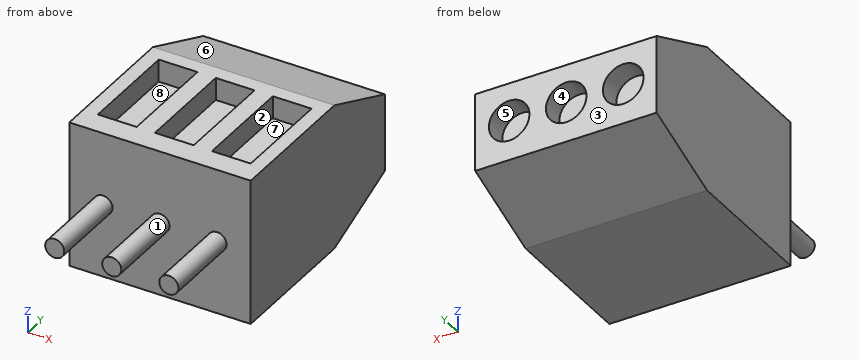
Autodesk Inventor part; units mm, degrees
ref_plane "YZ Plane" through (0, 0, 0) normal (1, 0, 0) x (0, 1, 0)
ref_plane "XZ Plane" through (0, 0, 0) normal (0, 1, 0) x (-1, 0, 0)
ref_plane "XY Plane" through (0, 0, 0) normal (0, 0, 1) x (1, 0, 0)
sketch "Sketch1" plane through (0, 0, 0) normal (1, 0, 0) x (0, 1, 0)
  line L0 (0, 3.25) -> (10, 3.25)
  line L1 (10, 3.25) -> (10, -3.25)
  line L2 (10, -3.25) -> (0, -3.25)
  line L3 (0, -3.25) -> (0, 3.25)
  line L4 (10, 1.6898) -> (6.2365, 3.25)
  line L5 (10, -1.7859) -> (6.2365, -3.25)
  point P0 (0, 0)
  dimension "d0" = 10
  dimension "d1" = 6.5
  dimension "d2" = 3.25
  dimension "d3" = 0
extrude "Extrusion1" add sketch "Sketch1" along normal mid plane 8.08 contours L0 L4 L1 L5 L2 L3
sketch "Sketch2" plane through (-4.04, 0, -3.25) normal (0, -1, 0) x (1, 0, 0)
  circle A0 centre (1.5, 3.25) radius 0.425
  line L0 (0, 0) -> (0, 6.5)
  point P0 (4.04, 3.25)
  dimension "d7" = 0.85
  dimension "d12" = 1.5
extrude "Extrusion2" add sketch "Sketch2" along normal blind 3.6
sketch "Sketch3" plane through (-4.04, 10, 1.6898) normal (0, 1, 0) x (1, 0, 0)
  circle A0 centre (1.4879, 1.6898) radius 0.904
  point P0 (4.04, 1.6898)
extrude "Extrusion3" cut sketch "Sketch3" against normal blind 1
sketch "Sketch4" plane through (-4.04, 0, 3.25) normal (0, 0, 1) x (1, 0, 0)
  line L0 (0.648, 5.5866) -> (2.3749, 5.5866)
  line L1 (2.3749, 5.5866) -> (2.3749, 1.0456)
  line L2 (2.3749, 1.0456) -> (0.648, 1.0456)
  line L3 (0.648, 1.0456) -> (0.648, 5.5866)
  point P0 (4.04, 0)
extrude "Extrusion4" cut sketch "Sketch4" against normal blind 1
pattern_linear "Rectangular Pattern1" count 3 spacing 2.54 along (1, 0, 0) of "Extrusion4", "Extrusion3", "Extrusion2"
properties part number "Screw_Terminal_3Pos"
CAD build for the part. Positions are in the model's coordinates, mm. Face numbers are marked on the shaded views. A direction names the side the tool comes from. Round coordinates to 2 decimals unless told otherwise and drop trailing zeros. Order: outer loops, then holes, each group sorted by start corner. A loop starts at its lowest first (then second) coordinate and runs counter-clockwise, first axis right, second up.
Q1. Slice it at A-A (z = 0). Write the cut outline in (x, y) (3 decimals), and give its area (3 significant figures).
Q2. Slice it at C-C (x = 1.25). Write the cut outline in (y, z).
Q3. Slice it at D-D (x = 2.5). Write the cut outline in (y, z).
Q4. Wall check: L1, parallel to X at y = 3.75, z = 2.75; L2, parallel to X at y = 9.6, z = 0; L3, parallel to Y at x = -3.5, z = 0.5. Give the ranges that are in metal, low to high.
Q5. Which spindle directions (+Z, -Z, +X, -X, +Y, -Y) get a long thin tool onto all of the face, cutting with end or side? Do the marked faces 1, 2, 3 and 4. Say none if no direction does.
Q6. Slice it at B-B (y = 2.5). Write the cut outline in (x, z).
Q7. Two-plate mould, pull along Y, no slides. Class the marked faces 5, 6, 7 and 8: pulls with the +Y half, pulls with the -Y half, needs draft (parallel to the pull), parting line crosses it, or undercut.
Q8. Drop flat-ended pins along their axis: pin 1 (1 mm diameter, centred on x = 2.5, z = -2, fed in from -Y); pin 2 (0.5 mm diameter, centred on x = 2.5, y = 3, fed in from +Z); pin 3 (1 mm diameter, centred on x = 0, y = -1, fed in from +Z) (3 decimals). Give the stop position or say it passes through.
Results below:
1. outline: (-4.04, 0) - (-2.965, 0) - (-2.965, -3.6) - (-2.115, -3.6) - (-2.115, 0) - (-0.425, 0) - (-0.425, -3.6) - (0.425, -3.6) - (0.425, 0) - (2.115, 0) - (2.115, -3.6) - (2.965, -3.6) - (2.965, 0) - (4.04, 0) - (4.04, 10) - (3.432, 10) - (3.432, 9) - (1.624, 9) - (1.624, 10) - (0.892, 10) - (0.892, 9) - (-0.916, 9) - (-0.916, 10) - (-1.648, 10) - (-1.648, 9) - (-3.456, 9) - (-3.456, 10) - (-4.04, 10) - close
1. area: 84.6 mm2
2. outline: (0, -3.25) - (6.24, -3.25) - (10, -1.79) - (10, 1.69) - (6.24, 3.25) - (0, 3.25) - close
3. outline: (-3.6, -0.42) - (0, -0.42) - (0, -3.25) - (6.24, -3.25) - (10, -1.79) - (10, -0.9) - (9, -0.9) - (9, 0.9) - (10, 0.9) - (10, 1.69) - (6.24, 3.25) - (5.59, 3.25) - (5.59, 2.25) - (1.05, 2.25) - (1.05, 3.25) - (0, 3.25) - (0, 0.42) - (-3.6, 0.42) - close
4. L1: x = -4.04 to -3.39, -1.67 to -0.85, 0.87 to 1.69, 3.41 to 4.04
4. L2: x = -4.04 to -3.46, -1.65 to -0.92, 0.89 to 1.62, 3.43 to 4.04
4. L3: y = 0 to 10
5. face 1: -Y
5. face 2: +Z
5. face 3: +Z, -Z, +X, -X, +Y
5. face 4: +Y
6. outline: (-4.04, -3.25) - (4.04, -3.25) - (4.04, 3.25) - (3.41, 3.25) - (3.41, 2.25) - (1.69, 2.25) - (1.69, 3.25) - (0.87, 3.25) - (0.87, 2.25) - (-0.85, 2.25) - (-0.85, 3.25) - (-1.67, 3.25) - (-1.67, 2.25) - (-3.39, 2.25) - (-3.39, 3.25) - (-4.04, 3.25) - close
7. face 5: needs draft
7. face 6: pulls with the +Y half
7. face 7: undercut
7. face 8: undercut
8. pin 1: stops at y = 0
8. pin 2: stops at z = 2.25
8. pin 3: stops at z = 0.425
